from build123d import *

# Parameters (mm, degrees)
SKETCH1_W                                            = 63.5
SKETCH1_H                                            = 12.7
CIRPATTERN1_COUNT                                    = 16
SKETCH24_R                                           = 19.05
BOSS_EXTRUDE1_DEPTH                                  = 12.7
CBORE_FOR_1_4_BINDING_HEAD_MACHINE_SCREW_D           = 7.14248
CBORE_FOR_1_4_BINDING_HEAD_MACHINE_SCREW_CBORE_D     = 14.2875
CBORE_FOR_1_4_BINDING_HEAD_MACHINE_SCREW_CBORE_DEPTH = 4.191


with BuildPart() as part:
    # Sketch1 → Revolve1 (revolve)
    with BuildSketch(Plane.XY):
        with Locations((82.55, 6.35)):
            Rectangle(SKETCH1_W, SKETCH1_H)
    revolve(axis=Axis((0, 58.205419954, 0), (0, -1, 0)))

    # Sketch20 → CBORE for 5_16 Binding Head Machine Scre (revolve, cut)
    with BuildSketch(Plane(origin=(65.1256, 12.7, 0), x_dir=(0, 0, 1), z_dir=(1, 0, 0))):
        Polygon((0, 0), (0, 12.7), (4.2164, 12.7), (4.2164, 10.16), (8.73125, 10.16), (8.73125, 0.15875), (8.89, 0), align=None)
    cbore_for_5_16_binding_head_machine_scre = revolve(axis=Axis((65.1256, 19.05, 0), (0, -1, 0)), mode=Mode.SUBTRACT)

    # CirPattern1: CBORE for 5_16 Binding Head Machine Scre ×16 about axis
    cirpattern1_axis = Axis((0, 0, 0), (0, 1, 0))
    for i in range(1, CIRPATTERN1_COUNT):
        add(cbore_for_5_16_binding_head_machine_scre.rotate(cirpattern1_axis, i * 360 / CIRPATTERN1_COUNT), mode=Mode.SUBTRACT)

    # Sketch24 → Boss-Extrude1 (add)
    with BuildSketch(Plane(origin=(0, 12.7, 0), x_dir=(1, 0, 0), z_dir=(0, 1, 0))):
        with Locations((-21.023532701, 105.692436214)):
            Circle(SKETCH24_R)
        with Locations((105.692436214, 21.023532701)):
            Circle(SKETCH24_R)
        with Locations((-105.692436214, -21.023532701)):
            Circle(SKETCH24_R)
        with Locations((21.023532701, -105.692436214)):
            Circle(SKETCH24_R)
    extrude(amount=-BOSS_EXTRUDE1_DEPTH)

    # CBORE for 1_4 Binding Head Machine Screw (through all)
    with Locations(Plane(origin=(0, 0, 0), x_dir=(-1, 0, 0), z_dir=(0, -1, 0))):
        with Locations((-21.023532701, -105.692436214), (-105.692436214, 21.023532701), (21.023532701, 105.692436214), (105.692436214, -21.023532701)):
            CounterBoreHole(CBORE_FOR_1_4_BINDING_HEAD_MACHINE_SCREW_D / 2, CBORE_FOR_1_4_BINDING_HEAD_MACHINE_SCREW_CBORE_D / 2, CBORE_FOR_1_4_BINDING_HEAD_MACHINE_SCREW_CBORE_DEPTH)


solid = part.part
Model file for the job. Use its own axes, mm. A direction names the side the tool comes from. Round coordinates to 2 decimals unless told otherwise and drop trailing zeros. Loops run counter-clockwise (first coordinate to the right, second up) from the corner with the lowest first, then second, coordinate; pieces in that order, holes last.
1. Band-saw the part on D-D, the plane z = 93. List the corners of the cut face in (x, y).
Check values:
outline: (-66.45, 0) - (66.45, 0) - (66.45, 12.7) - (-66.45, 12.7) - close
2. Mould opens along X. For faces 1 (the flat face through (2, 12.7, -54)), 2 (the cylindrical face through (-48.31, 1.29, 49.61)) say: +X half, -X half, draft (parallel to the pull), parting line (faces both ways), or undercut.
Check values:
face 1: draft
face 2: undercut
3. Wall check: probe 1 along Z at (x, y) = (0, 7); probe 2 along Z at (x, y) = (-0.5, 11); probe 3 along X at (y, z) = (9.75, -20). Give the ranges that are in metal, low to high.
Check values:
probe 1: z = -114.3 to -73.86, -56.39 to -50.8, 50.8 to 56.39, 73.86 to 114.3
probe 2: z = -114.3 to -73.84, -56.41 to -50.8, 50.8 to 56.41, 73.84 to 114.3
probe 3: x = -112.54 to -67.38, -52.96 to -46.7, 46.7 to 52.96, 67.38 to 102.27, 109.11 to 124.71
4. Band-saw the part on B-B, the plane z = 0. List the corners of the cut face in (x, y), and give its area (3 significant figures).
Check values:
outline: (-114.3, 0) - (-69.34, 0) - (-69.34, 2.54) - (-73.86, 2.54) - (-73.86, 12.54) - (-74.02, 12.7) - (-114.3, 12.7) - close; (-60.91, 0) - (-50.8, 0) - (-50.8, 12.7) - (-56.24, 12.7) - (-56.39, 12.54) - (-56.39, 2.54) - (-60.91, 2.54) - close; (50.8, 0) - (60.91, 0) - (60.91, 2.54) - (56.39, 2.54) - (56.39, 12.54) - (56.24, 12.7) - (50.8, 12.7) - close; (69.34, 0) - (114.3, 0) - (114.3, 12.7) - (74.02, 12.7) - (73.86, 12.54) - (73.86, 2.54) - (69.34, 2.54) - close
area: 1,220 mm2
5. Drop flat-ended pins along their axis: P1, Ø6, axis at y = 1.5, z = 14, coming from the -X side; P2, Ø11, axis at x = 46.05, z = 46.05, coming from the +Y side; P3, Ø2, axis at y = 4, z = -99.5, coming from the -X side. Give the stop position or say it passes through.
Check values:
P1: stops at x = -124.31
P2: stops at y = 2.54
P3: stops at x = -57.98
6. Band-saw the part on C-C, the plane y = 10. Count the separate pieces of the cut face and the enclosed holes in it, and give its area (3 significant figures).
Check values:
separate pieces: 1
enclosed holes: 21
area: 30,300 mm2
7. Band-saw the part on A-A, the plane x = 0. List the corners of the cut face in (y, z), and give its area (3 significant figures).
Check values:
outline: (0, -114.3) - (12.7, -114.3) - (12.7, -74.02) - (12.54, -73.86) - (2.54, -73.86) - (2.54, -69.34) - (0, -69.34) - close; (0, -60.91) - (2.54, -60.91) - (2.54, -56.39) - (12.54, -56.39) - (12.7, -56.24) - (12.7, -50.8) - (0, -50.8) - close; (0, 50.8) - (12.7, 50.8) - (12.7, 56.24) - (12.54, 56.39) - (2.54, 56.39) - (2.54, 60.91) - (0, 60.91) - close; (0, 69.34) - (2.54, 69.34) - (2.54, 73.86) - (12.54, 73.86) - (12.7, 74.02) - (12.7, 114.3) - (0, 114.3) - close
area: 1,220 mm2
8. Tool access for faces 3 (the cylindrical face through (-26.436, 7.611, 68.767)), 4 (the cylindrical face through (48.31, 1.29, -49.61)): list every direction of +Z, -Z, +X, -X, +Y, -Y with a clear straight run to the whole face (end or side of a thin tool).
Check values:
face 3: +Y
face 4: +Y, -Y
